Geometry check sheet. Reference: the model listing, model coordinates, mm. Face numbers are marked on the shaded views. Give positions to 0.01 mm unless a question says otherwise; leave off trailing zeros. Loops run counter-clockwise (first coordinate to the right, second up) from the corner with the lowest first, then second, coordinate; pieces in that order, holes last.
```python
from build123d import *

# Parameters (mm, degrees)
F1_START      = 20
F0_W          = 10
F0_H          = 260
F1_DEPTH      = 260
F2_DEPTH      = 300
F3_R          = 4.5
F4_DEPTH      = 15.001
F4_DEPTH_BACK = 275.001
F5_SIZE       = 5
F7_DEPTH      = 50.001
F8_R          = 5


with BuildPart() as f1:
    # F0 (on Top) → F1 (new body)
    with BuildSketch(Plane.XY.offset(F1_START)):
        with Locations((45, 145)):
            Rectangle(F0_W, F0_H)
    extrude(amount=F1_DEPTH)

    # F0 (on Top) → F2 (join)
    with BuildSketch(Plane.XY):
        Polygon((45, 290), (0, 290), (0, 285), (40, 275), (50, 275), (90, 285), (90, 290), align=None)
        Polygon((50, 15), (40, 15), (0, 5), (0, 0), (45, 0), (90, 0), (90, 5), align=None)
    extrude(amount=F2_DEPTH)

    # F3 (on face) → F4 (cut, two sides)
    with BuildSketch(Plane(origin=(0, 15, 0), x_dir=(-1, 0, 0), z_dir=(0, 1, 0))) as f4_sk:
        with Locations((-45, 290)):
            Circle(F3_R)
        with Locations((-45, 10)):
            Circle(F3_R)
    extrude(amount=-F4_DEPTH, mode=Mode.SUBTRACT)
    extrude(f4_sk.sketch, amount=F4_DEPTH_BACK, mode=Mode.SUBTRACT)

    # F5
    f5_edges = [f1.edges().sort_by_distance(p)[0] for p in [
        (50, 275, 150),
        (40, 275, 150),
        (40, 15, 150),
        (50, 15, 150),
    ]]
    chamfer(f5_edges, length=F5_SIZE)

    # F6 (on face) → F7 (cut, through all)
    with BuildSketch(Plane.YZ.offset(50)):
        Polygon((135, 260), (49.1421356237, 260), (135, 174.1421356237), align=None)
        Polygon((240.8578643763, 260), (155, 260), (155, 174.1421356237), align=None)
        Polygon((250, 160), (250, 240.8578643763), (169.1421356237, 160), align=None)
        Polygon((250, 59.1421356237), (250, 140), (169.1421356237, 140), align=None)
        Polygon((155, 125.8578643763), (155, 40), (240.8578643763, 40), align=None)
        Polygon((135, 125.8578643763), (49.1421356237, 40), (135, 40), align=None)
        Polygon((120.8578643763, 140), (40, 140), (40, 59.1421356237), align=None)
        Polygon((40, 160), (120.8578643763, 160), (40, 240.8578643763), align=None)
        Polygon((155, 145.8578643763), (155, 154.1421356237), (149.1421356237, 160), (140.8578643763, 160), (135, 154.1421356237), (135, 145.8578643763), (140.8578643763, 140), (149.1421356237, 140), align=None)
    extrude(amount=-F7_DEPTH, mode=Mode.SUBTRACT)

    # F8
    f8_edges = [f1.edges().sort_by_distance(p)[0] for p in [
        (45, 240.857864, 260),
        (45, 155, 260),
        (45, 155, 174.142136),
        (45, 250, 240.857864),
        (45, 250, 160),
        (45, 169.142136, 160),
        (45, 250, 140),
        (45, 250, 59.142136),
        (45, 169.142136, 140),
        (45, 155, 125.857864),
        (45, 240.857864, 40),
        (45, 155, 40),
        (45, 135, 125.857864),
        (45, 135, 40),
        (45, 49.142136, 40),
        (45, 40, 59.142136),
        (45, 40, 140),
        (45, 120.857864, 140),
        (45, 40, 160),
        (45, 40, 240.857864),
        (45, 120.857864, 160),
        (45, 135, 174.142136),
        (45, 49.142136, 260),
        (45, 135, 260),
        (45, 135, 145.857864),
        (45, 135, 154.142136),
        (45, 140.857864, 160),
        (45, 149.142136, 160),
        (45, 155, 154.142136),
        (45, 155, 145.857864),
        (45, 149.142136, 140),
        (45, 140.857864, 140),
    ]]
    fillet(f8_edges, radius=F8_R)


solid = f1.part
```
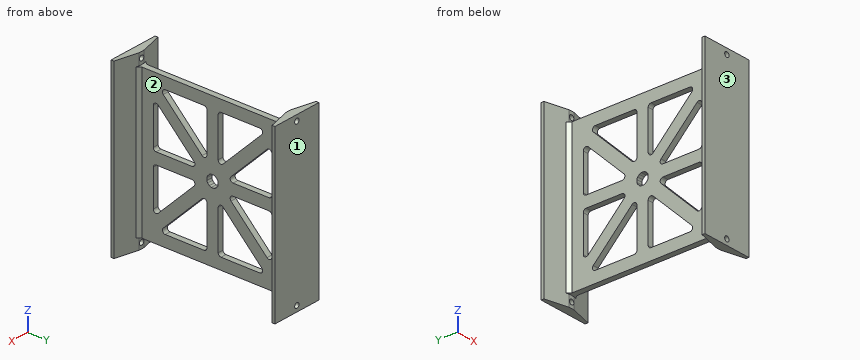
1) Sectioned sample at B-B on x = 45. Count the separate pieces of the cut face and the enclosed holes in it, plus the area to 3 significant figures.
2) Sectioned sample at C-C on x = 72.5. Enter the section's corners in (y, z) (3 decimals).
3) Sectioned sample at A-A on z = 10. Enter the section's corners in (x, y).
4) Sectioned sample at D-D on z = 127. Enter the section's corners in (x, y).
5) Mould release check, pull along Y, two halves, no side actions. Record for the marked faces 1, 2 and 3: +Y half, -Y half, draft (parallel to the pull), parting line (faces both ways), or undercut.
6) Depth check by flat-ended pin: P1, Ø11, axis at x = 43, y = 91.5, coming from the +Z side; P2, Ø5, axis at x = 45, y = 219, coming from the -Z side; P3, Ø5, axis at y = 73, z = 239.5, coming from the +X side. Enter the tip coordinate at first touch or a pass-through.
7) Scan lines: line 1 along Z through (x, y) = (45, 285); line 2 along Z through (x, y) = (44, 221); line 3 along Y through (x, z) = (44.5, 43). Record each from-to range of solid material in increasing order.
Determined:
1. separate pieces: 5
1. enclosed holes: 9
1. area: 48,500 mm2
2. outline: (0, 0) - (9.375, 0) - (9.375, 300) - (0, 300) - close; (280.625, 0) - (290, 0) - (290, 300) - (280.625, 300) - close
3. outline: (0, 0) - (40.5, 0) - (40.5, 15) - (40, 15) - (0, 5) - close; (0, 285) - (40, 275) - (40.5, 275) - (40.5, 290) - (0, 290) - close; (49.5, 0) - (90, 0) - (90, 5) - (50, 15) - (49.5, 15) - close; (49.5, 275) - (50, 275) - (90, 285) - (90, 290) - (49.5, 290) - close
4. outline: (0, 0) - (90, 0) - (90, 5) - (54.85, 13.79) - (50, 20) - (50, 40) - (40, 40) - (40, 20) - (35.15, 13.79) - (0, 5) - close; (0, 285) - (35.15, 276.21) - (40, 270) - (40, 250) - (50, 250) - (50, 270) - (54.85, 276.21) - (90, 285) - (90, 290) - (0, 290) - close; (40, 107.86) - (50, 107.86) - (50, 182.14) - (40, 182.14) - close
5. face 1: +Y half
5. face 2: undercut
5. face 3: -Y half
6. P1: stops at z = 280
6. P2: stops at z = 20
6. P3: stops at x = 50
7. line 1: z = 0 to 5.5, 14.5 to 285.5, 294.5 to 300
7. line 2: z = 20 to 40, 59.86 to 88.14, 140 to 160, 211.86 to 240.14, 260 to 280
7. line 3: y = 0 to 56.63, 134.58 to 155.42, 233.37 to 290
